CAD build for the part. Positions are in the model's coordinates, mm. A direction names the side the tool comes from. Round coordinates to 2 decimals unless told otherwise and drop trailing zeros. Write each loop counter-clockwise with the first axis right and the second up, starting at its lowest first coordinate (ties: lowest second). Pieces come first, ordered by that corner, then holes. Notation, with made-up numbers: (-11.75, 52) - (7.25, 52) arc R14 cw to (7.25, 62) - close; hole circle Ø11 at (-29, 28.5). An arc over 180 degrees is marked (long way). Put each result on its own line as item: value. Start each with the question number.
Item 1: Cut at C-C (y = 7). Give the cut face in (x, z), and give its area (3 significant figures).
Item 2: Cut at B-B (z = 1.5). Give the cut face in (x, y), and give its area (3 significant figures).
Item 3: 3-axis set-ups, long thin cutter, end or side, ignore diameter. For faces 1 (the flat face through (0, 11, -5)), 2 (the flat face through (18, 1, 0)), 3 (the flat face through (27, 11, 0)): which of +Z, -Z, +X, -X, +Y, -Y reach the whole face in a straight line?
Item 4: Drill centre lines: line 1 (X direction, y = 0.4, z = 0); line 2 (Z direction, x = -22, y = 11.25); line 3 (X direction, y = 4.75, z = -0.5). Where is each one in solid material? Low to high. Write a range as from..to.
Item 5: Mould opens along Z. For faces 4 (the flat face through (0, 11, -7)), 5 (the cylindrical face through (-22.476, 0.986, -0.217)), 6 (the flat face through (21.5, 2, -1.2)), 7 (the flat face through (-27, 11, 0)) say: released by +Z, released by -Z, zero draft, split by the parting line, or undercut.
Item 6: Pin check, flat tip, straight feed: pin 1 Ø2 at (x, z) = (22, -1.5) entering from +Y. Stop position of the tip, or through.
Item 7: Cut at D-D (x = 4). Give the cut face in (y, z).
Item 8: Cut at A-A (x = 21.5). Give the cut face in (y, z).
```python
from build123d import *

# Parameters (mm, degrees)
SKETCH3_W           = 54
SKETCH3_H           = 14
SKETCH3_W_2         = 50
SKETCH3_H_2         = 10
BOSS_EXTRUDE1_DEPTH = 22
SKETCH4_W           = 7
SKETCH4_H           = 10
SKETCH4_R           = 1
BOSS_EXTRUDE2_DEPTH = 2


with BuildPart() as part:
    # Sketch3 → Boss-Extrude1 (new body)
    with BuildSketch(Plane(origin=(0, 0, 0), x_dir=(1, 0, 0), z_dir=(0, 1, 0))):
        Rectangle(SKETCH3_W, SKETCH3_H)
        Rectangle(SKETCH3_W_2, SKETCH3_H_2, mode=Mode.SUBTRACT)
    extrude(amount=BOSS_EXTRUDE1_DEPTH)

    # Sketch4 → Boss-Extrude2 (add)
    # profile 1 of 2: a face of its own
    with BuildSketch(Plane(origin=(0, 0, 0), x_dir=(1, 0, 0), z_dir=(0, 1, 0))):
        with Locations((-21.5, 0)):
            Rectangle(SKETCH4_W, SKETCH4_H)
        with Locations(Location((-21.5, 0, 0), (0, 0, 270))):
            Circle(SKETCH4_R, mode=Mode.SUBTRACT)
    # profile 2 of 2: a face of its own
    with BuildSketch(Plane(origin=(0, 0, 0), x_dir=(1, 0, 0), z_dir=(0, 1, 0))):
        with Locations((21.5, 0)):
            Rectangle(SKETCH4_W, SKETCH4_H)
        with Locations(Location((21.5, 0, 0), (0, 0, 270))):
            Circle(SKETCH4_R, mode=Mode.SUBTRACT)
    extrude(amount=BOSS_EXTRUDE2_DEPTH)


solid = part.part
```
Output values:
1. outline: (-27, -7) - (27, -7) - (27, 7) - (-27, 7) - close; hole (-25, -5) - (25, -5) - (25, 5) - (-25, 5) - close
1. area: 256 mm2
2. outline: (-27, 0) - (-18, 0) - (-18, 2) - (-25, 2) - (-25, 22) - (-27, 22) - close; (18, 0) - (27, 0) - (27, 22) - (25, 22) - (25, 2) - (18, 2) - close
2. area: 116 mm2
3. face 1: +Y
3. face 2: +Y, -Y
3. face 3: +Z, -Z, +X, +Y, -Y
4. line 1: -27..-22.5, -20.5..-18, 18..20.5, 22.5..27
4. line 2: -7..-5, 5..7
4. line 3: -27..-25, 25..27
5. face 4: released by -Z
5. face 5: undercut
5. face 6: undercut
5. face 7: zero draft
6. pin 1: y = 2
7. outline: (0, -7) - (22, -7) - (22, -5) - (0, -5) - close; (0, 5) - (22, 5) - (22, 7) - (0, 7) - close
8. outline: (0, -7) - (22, -7) - (22, -5) - (2, -5) - (2, -1) - (0, -1) - close; (0, 1) - (2, 1) - (2, 5) - (22, 5) - (22, 7) - (0, 7) - close
